Read the model definition and answer for the solid it produces. Units are mm, in the model's axes. Face numbers are marked on the shaded views. Coordinates: 2 decimals unless noted, no trailing zeros. Write each loop counter-clockwise with the first axis right and the second up, starting at its lowest first coordinate (ties: lowest second). Pieces come first, ordered by that corner, then holes.
1) Find the intervals of material crossed by line 1 (Z direction, x = -0.5, y = 60); line 2 (Y direction, x = 10, z = -16.5); line 3 (Y direction, x = -16, z = -34), in increasing order.
2) Each of these flat-tipped pins is pushed along its axis until it touches: pin 1 Ø1 at (x, z) = (-18.5, -3) entering from +Y; pin 2 Ø4 at (x, y) = (-4, 18) entering from +Z; pin 3 Ø1.5 at (y, z) = (28, -7) entering from +X. Where does it stop, or does it pass through?
3) The part is cut by section A-A (y = 74). Determine the outline of the cut face in (x, z).
4) Determine the mould class of the marked faces 1, 2 and 3 for opening direction X: +X half, -X half, draft (parallel to the pull), parting line (faces both ways), or undercut.
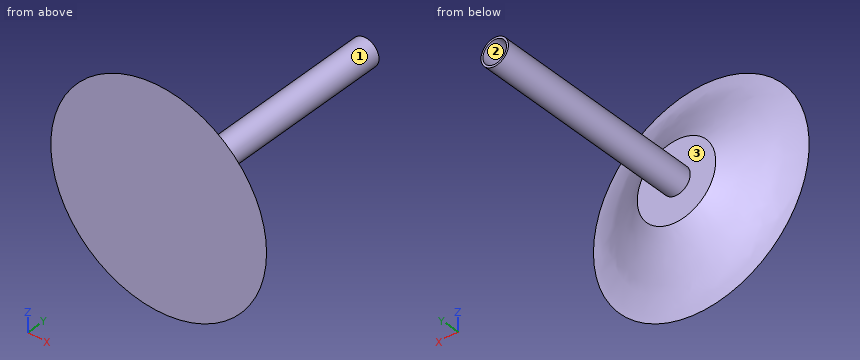
from build123d import *

# Parameters (mm, degrees)
F2_R     = 7
F3_DEPTH = 110
F4_T     = -1


with BuildPart() as f1:
    # F0 (on Top) → F1 (revolve)
    with BuildSketch(Plane.XY):
        with BuildLine():
            Line((20, 15), (0, 15))
            Line((0, 15), (0, 0))
            Line((0, 0), (55, 0))
            add(Edge.make_bspline(
                [(20, 15), (26.4091145129, 11.0259934035), (39.2875073258, 5.0952762992), (46.8235665253, 1.1879222139), (55, 0)],
                knots=[0, 0, 0, 0, 0.5215307658, 1, 1, 1, 1], degree=3))
        make_face()
    revolve(axis=Axis((0, 7.5, 0), (0, -1, 0)))

    # F2 (on face) → F3 (join)
    with BuildSketch(Plane(origin=(0, 15, 0), x_dir=(-1, 0, 0), z_dir=(0, 1, 0))):
        Circle(F2_R)
    extrude(amount=F3_DEPTH)

    # F4
    f4_openings = [f1.faces().sort_by_distance(p)[0] for p in [
        (0, 125, 0),
    ]]
    offset(amount=F4_T, openings=f4_openings, kind=Kind.INTERSECTION)


solid = f1.part
Reported:
1. line 1: z = -6.98 to -5.98, 5.98 to 6.98
1. line 2: y = 0 to 1, 14 to 15
1. line 3: y = 0 to 1, 4.67 to 5.78
2. pin 1: stops at y = 15
2. pin 2: stops at z = 6.71
2. pin 3: stops at x = 3.15
3. outline: circle Ø14 at (0, 0); hole circle Ø12 at (0, 0)
4. face 1: parting line
4. face 2: undercut
4. face 3: draft
